For this review, use the dimensioned drawing (mm, ordinates from the lowest corner) and the shaded views. A direction names the side the tool comes from. Give positions to 0.01 mm unless a question says otherwise; leave off trailing zeros. Write each loop counter-clockwise with the first axis right and the second up, starting at its lowest first coordinate (ties: lowest second). Pieces come first, ordered by that corner, then holes.
1) Wall thickness on line 1 along X through (y, z) = (1.55, 6.35); line 2 along Z through (x, y) = (17.5, 1.7); line 3 along X through (y, z) = (1, 6.35): over which ranges is each line inside the solid? List them lowest first.
2) Draft analysis for pull direction Z (two halves, no side actions). For the marked faces 3, 4 and 5, state which applies: pulls with the +Z half, pulls with the -Z half, needs draft (parallel to the pull), parting line crosses it, or undercut.
3) We need section B-B on x = 5.25. Give the boundary of the cut face in (y, z).
4) We need section C-C on y = 0.55. Give the boundary of the cut face in (x, z).
5) Machinability: for the marked faces 1 and 2, which of the approach directions +Z, -Z, +X, -X, +Y, -Y give a long, thin tool a straight path to every point of the face, cutting with its end or side? Answer none if there is none.
6) We need section D-D on z = 5.5. Give the boundary of the cut face in (x, y).
7) We need section A-A on y = 1.65. Give the number of separate pieces and of enclosed holes in the cut face, and give its area (3 significant figures).
8) For P1, Ø1.4, axis at x = 19, y = 2, coming from the -Z side; P2, Ø1, axis at x = 5.5, y = 0.5, coming from the +Z side, all flat-tipped, find the tip position at first contact; note any pin that passes through.
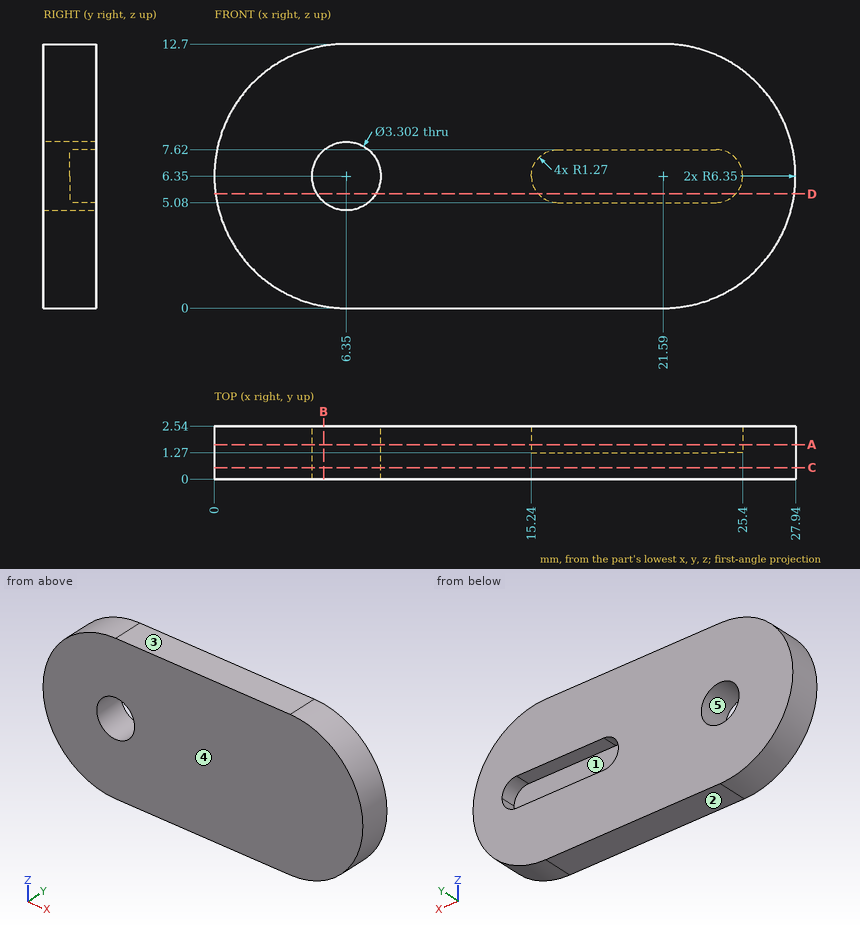
Results list:
1. line 1: x = 0 to 4.7, 8 to 15.24, 25.4 to 27.94
1. line 2: z = 0 to 5.08, 7.62 to 12.7
1. line 3: x = 0 to 4.7, 8 to 27.94
2. face 3: pulls with the +Z half
2. face 4: needs draft
2. face 5: undercut
3. outline: (0, 0.1) - (2.54, 0.1) - (2.54, 5.12) - (0, 5.12) - close; (0, 7.58) - (2.54, 7.58) - (2.54, 12.6) - (0, 12.6) - close
4. outline: (6.35, 0) - (21.59, 0) arc R6.35 ccw to (21.59, 12.7) - (6.35, 12.7) arc R6.35 ccw to start; hole circle Ø3.3 at (6.35, 6.35)
5. face 1: +Y
5. face 2: -Z, +X, -X, +Y, -Y
6. outline: (0.06, 0) - (4.93, 0) - (4.93, 2.54) - (0.06, 2.54) - close; (7.77, 0) - (27.88, 0) - (27.88, 2.54) - (25.07, 2.54) - (25.07, 1.27) - (15.57, 1.27) - (15.57, 2.54) - (7.77, 2.54) - close
7. separate pieces: 1
7. enclosed holes: 2
7. area: 287 mm2
8. P1: stops at z = 0
8. P2: stops at z = 12.69
